```python
from build123d import *

# Parameters (mm, degrees)
CROQUIS1_R              = 21
SALIENTE_EXTRUIR1_DEPTH = 40
SALIENTE_EXTRUIR2_DEPTH = 40
SALIENTE_EXTRUIR3_REACH = 77.493
CROQUIS3_R              = 13.5
CROQUIS3_R_2            = 10
CROQUIS7_R              = 8.227269221
CROQUIS7_R_2            = 6
CORTAR_EXTRUIR6_DEPTH   = 6
CROQUIS8_R              = 6
CORTAR_EXTRUIR7_DEPTH   = 72.223648425
CORTAR_EXTRUIR8_START   = -25
CORTAR_EXTRUIR8_DEPTH   = 25
CROQUIS12_R             = 9.55
CORTAR_EXTRUIR9_DEPTH   = 5.5


with BuildPart() as part:
    # Croquis1 → Saliente-Extruir1 (new body)
    with BuildSketch(Plane(origin=(0, 0, 0), x_dir=(1, 0, 0), z_dir=(0, 1, 0))):
        with Locations(Location((0, 0, 0), (0, 0, 270))):
            Circle(CROQUIS1_R)
    extrude(amount=SALIENTE_EXTRUIR1_DEPTH)

    # Croquis2 → Saliente-Extruir2 (add)
    with BuildSketch(Plane(origin=(0, 0, 0), x_dir=(1, 0, 0), z_dir=(0, 1, 0))):
        with BuildLine():
            Line((53.975127576, 8.110971331), (53.975127576, -11.889028669))
            Line((53.975127576, -11.889028669), (3.613793412, -20.686722727))
            ThreePointArc((3.613793412, -20.686722727), (20.98607707, -0.764571273), (5.109545014, 20.368911354))
            Line((5.109545014, 20.368911354), (53.975127576, 8.110971331))
        make_face()
    extrude(amount=SALIENTE_EXTRUIR2_DEPTH)

    # Croquis3 → Saliente-Extruir3 (add, up to next)
    with BuildSketch(Plane(origin=(5.109545014, 0, -20.368911354), x_dir=(-0.9699481597219111, 0, -0.24331166731597212), z_dir=(0.2433116673159721, 0, -0.969948159721911)), mode=Mode.PRIVATE) as saliente_extruir3_sk1:
        with Locations((0, 20)):
            Circle(CROQUIS3_R)
        with Locations((0, 20)):
            Circle(CROQUIS3_R_2, mode=Mode.SUBTRACT)
    saliente_extruir3_tool1 = extrude(saliente_extruir3_sk1.sketch, amount=-SALIENTE_EXTRUIR3_REACH, mode=Mode.PRIVATE) - part.part
    add(saliente_extruir3_tool1.solids().sort_by_distance((17.833482, 20, -17.177109))[0])

    # Croquis7 → Cortar-Extruir6 (cut)
    with BuildSketch(Plane.XZ):
        with Locations(Location((0, 0, 0), (0, 0, 270))):
            Circle(CROQUIS7_R)
        with Locations(Location((0, 0, 0), (0, 0, 270))):
            Circle(CROQUIS7_R_2, mode=Mode.SUBTRACT)
    extrude(amount=-CORTAR_EXTRUIR6_DEPTH, mode=Mode.SUBTRACT)

    # Croquis8 → Cortar-Extruir7 (cut, through all)
    with BuildSketch(Plane.XZ):
        with Locations(Location((0, 0, 0), (0, 0, 270))):
            Circle(CROQUIS8_R)
    extrude(amount=-CORTAR_EXTRUIR7_DEPTH, mode=Mode.SUBTRACT)

    # Croquis10 → Cortar-Extruir8 (cut)
    with BuildSketch(Plane(origin=(0, 40, 0), x_dir=(1, 0, 0), z_dir=(0, 1, 0)).offset(CORTAR_EXTRUIR8_START)):
        with BuildLine():
            Line((-5.995438853, 0.23390802), (-11.37823559, 0.424457107))
            Line((-11.37823559, 0.424457107), (-11.767631672, -10.575542893))
            Line((-11.767631672, -10.575542893), (30.232368328, -12.062327932))
            Line((30.232368328, -12.062327932), (30.62176441, -1.062327932))
            Line((30.62176441, -1.062327932), (5.996971268, -0.190619027))
            ThreePointArc((5.996971268, -0.190619027), (-0.212264906, -5.996244125), (-5.995438853, 0.23390802))
        make_face()
        with BuildLine():
            Line((-10.988839509, 11.424457107), (-11.37823559, 0.424457107))
            Line((-11.37823559, 0.424457107), (-5.995438853, 0.23390802))
            ThreePointArc((-5.995438853, 0.23390802), (0.116976243, 5.998859605), (6, 0))
            ThreePointArc((6, 0), (5.999242769, -0.095321543), (5.996971268, -0.190619027))
            Line((5.996971268, -0.190619027), (30.62176441, -1.062327932))
            Line((30.62176441, -1.062327932), (31.011160491, 9.937672068))
            Line((31.011160491, 9.937672068), (-10.988839509, 11.424457107))
        make_face()
    extrude(amount=CORTAR_EXTRUIR8_DEPTH, mode=Mode.SUBTRACT)

    # Croquis12 → Cortar-Extruir9 (cut)
    with BuildSketch(Plane(origin=(0, 15, 0), x_dir=(1, 0, 0), z_dir=(0, 1, 0))):
        with Locations(Location((0, 0, 0), (0, 0, 270))):
            Circle(CROQUIS12_R)
    extrude(amount=-CORTAR_EXTRUIR9_DEPTH, mode=Mode.SUBTRACT)

    # Croquis4 → Revolución1 (revolve)
    with BuildSketch(Plane(origin=(5.1, 0, 0), x_dir=(0, 0, -1), z_dir=(1, 0, 0))):
        Polygon((20.368911354, 6.46), (14.136824823, 7.062482259), (14.475882844, 10.569704081), (20.368911354, 10), (44.36703003, 7.68), (44.36703003, 4.14), align=None)
    revolve(axis=Axis((5.1, 20, -20.368911354), (0, -0.09622563251762795, -0.9953595469209016)))


solid = part.part
```
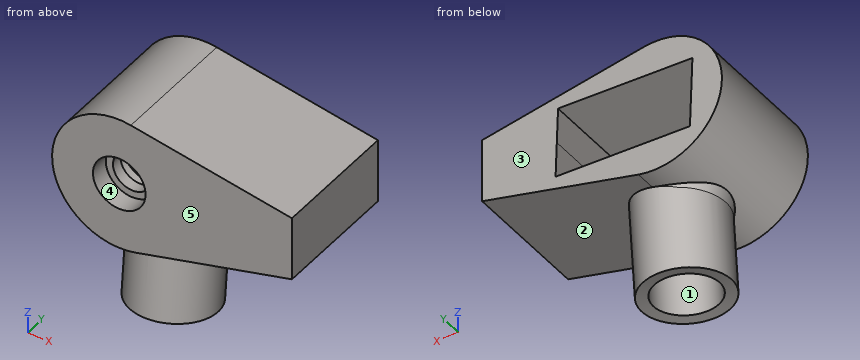
Geometry check sheet. Reference: the model listing, model coordinates, mm. Face numbers are marked on the shaded views. A direction names the side the tool comes from. Give positions to 0.01 mm unless a question says otherwise; leave off trailing zeros. Order: outer loops, then holes, each group sorted by start corner. A loop starts at its lowest first (then second) coordinate and runs counter-clockwise, first axis right, second up. Notation, with made-up numbers: (39, -29.5) - (69, -29.5) arc R18 ccw to (69, 0.5) - close; hole circle Ø4 at (44, 19.5). An arc over 180 degrees is marked (long way). Answer in a Markdown table with one row per item. Add a question column.
Q1. Mould release check, pull along X, two halves, no side actions. Record for the marked faces 1, 2 and 3: pulls with the +X half, pulls with the -X half, needs draft (parallel to the pull), parting line crosses it, or undercut.
Q2. Cross-section at A-A, the plane y = 35. Enter the section's corners in (x, z), then the cut area to 3 significant figures.
Q3. Cross-section at D-D, the plane z = 17. Enter the section's corners in (x, y), then the cut area to 3 significant figures.
Q4. Material ranges on probe 1 along X at (y, z) = (6.85, 0); probe 2 along X at (y, z) = (1.5, 0); probe 3 along Z at (x, y) = (21, 23), recorded low to high. Write a range as from..to.
Q5. Cross-section at C-C, the plane x = 47. Enter the section's corners in (y, z), then the cut area to 3 significant figures.
Q6. Cross-section at B-B, the plane z = 7. Enter the section's corners in (x, y).
Q7. Tool access check on the marked faces 4 and 5. Record the directions out of +Z, -Z, +X, -X, +Y, -Y that give a thin tool (end or side, any length) a straight path to the whole face; none if there is none.
Q8. Gauge pin test, flat ends, axial feed: pin 1 (3 mm diameter, centred on x = 32, y = 32.5, fed in from +Z); pin 2 (3 mm diameter, centred on x = 33.5, y = 20, fed in from +Z); pin 3 (12 mm diameter, centred on y = 6.5, z = -12, fed in from -X). Record the tip position at first contact, or that the pin passes through.
Check values:
| question | item | result |
|---|---|---|
| 1 | face 1 | undercut |
| 1 | face 2 | pulls with the +X half |
| 1 | face 3 | needs draft |
| 2 | outline | (3.61, 20.69) arc R21 ccw (long way) to (5.11, -20.37) - (53.98, -8.11) - (53.98, 11.89) - close; hole (-11.77, 10.58) - (-10.99, -11.42) - (31.01, -9.94) - (30.23, 12.06) - close |
| 2 | area | 1,470 mm^2 |
| 3 | outline | (-12.33, 0) - (24.72, 0) - (24.72, 40) - (-12.33, 40) - close |
| 3 | area | 1,480 mm^2 |
| 4 | probe 1 | x = -21..-6, 6..53.98 |
| 4 | probe 2 | x = -21..-8.23, 8.23..53.98 |
| 4 | probe 3 | z = -16.38..-10.29, 11.74..17.65 |
| 5 | outline | (0, -9.86) - (40, -9.86) - (40, 13.11) - (0, 13.11) - close |
| 5 | area | 919 mm^2 |
| 6 | outline | (-19.8, 0) - (-4.32, 0) - (-4.32, 6) - (4.32, 6) - (4.32, 0) - (53.98, 0) - (53.98, 40) - (30.41, 40) - (30.41, 15) - (6.5, 15) - (6.5, 9.5) - (-6.5, 9.5) - (-6.5, 15) - (-11.64, 15) - (-11.64, 40) - (-19.8, 40) - close |
| 7 | face 4 | -Y |
| 7 | face 5 | +Z, -Z, +X, -X, -Y |
| 8 | pin 1 | stops at z = 15.99 |
| 8 | pin 2 | stops at z = 15.73 |
| 8 | pin 3 | stops at x = -20.12 |
